For this review, take the finished solid that the model builds, in its own axes (mm). A direction names the side the tool comes from. Round coordinates to 2 decimals unless told otherwise and drop trailing zeros. Order: outer loops, then holes, each group sorted by start corner. A loop starts at its lowest first (then second) coordinate and runs counter-clockwise, first axis right, second up. Notation, with made-up numbers: (-37, -37.75) -> (4, -37.75) arc R18 cw to (4, -6.75) -> close; hole circle Ø4 at (55, -3.5). An arc over 180 degrees is marked (long way). Use a Markdown table: item, result. Add a question column.
1) Draft analysis for pull direction Y (two halves, no side actions). For faces 5 (the face through (9, -2.54, 64)), 6 (the face through (10, 4, 25.4)), 7 (the face through (14.188, 4, 15)), state which applies: pulls with the +Y half, pulls with the -Y half, needs draft (parallel to the pull), parting line crosses it, or undercut.
2) Machinability: for faces 1 (the face through (13.31, 5.03, 12.52)), 2 (the face through (19.05, -1, 56)), 3 (the face through (10, 4, 30.48)), 4 (the face through (6.568, 4, 15)), which of the approach directions +Z, -Z, +X, -X, +Y, -Y give a long, thin tool a straight path to every point of the face, cutting with its end or side? Answer none if there is none.
3) Consider section D-D (y = -1.25). State the section outline as (x, z) points (3 decimals), plus the area to 3 significant figures.
4) Wall thickness on line 1 along X through (y, z) = (3.81, 18); line 2 along Y through (x, z) = (13, 40); line 3 along Y through (x, z) = (10.25, 23.5): over which ranges is each line inside the solid? List them lowest first. Write a range as [from, to].
5) Clearance check with flat-ended pins moving along their axes: P1, Ø5, axis at x = 11.5, y = 3.5, coming from the -Z side; P2, Ø4, axis at x = 10.38, y = 3.81, coming from the -Z side; P3, Ø4, axis at x = 13.5, y = 5.5, coming from the +Z side; P4, Ø10, axis at x = 15.5, z = 92, coming from the +Y side. State where each tip first meets the part, or that it passes through.
6) Consider section A-A (z = 26.5). State the section outline as (x, y) points, plus the area to 3 significant figures.
7) Consider section C-C (x = 11). State the section outline as (y, z) points, plus the area to 3 significant figures.
8) Consider section B-B (y = 3.81). State the section outline as (x, z) points.
```python
from build123d import *

# Parameters (mm, degrees)
F1_DEPTH = 2.54
F2_W     = 7.62
F2_H     = 30.48
F3_DEPTH = 7.62
F4_R     = 3.175
F5_DEPTH = 25.4


with BuildPart() as f1:
    # F0 (on Front) → F1 (new body)
    with BuildSketch(Plane.XZ):
        Polygon((0, 114.3), (0, 0), (19.05, 0), (19.05, 114.3), (9.525, 127), align=None)
    extrude(amount=F1_DEPTH)

    # F2 (on face) → F3 (join)
    with BuildSketch(Plane(origin=(0, 0, 0), x_dir=(-1, 0, 0), z_dir=(0, 1, 0))):
        with Locations((-10.377643, 15.24)):
            Rectangle(F2_W, F2_H)
    extrude(amount=F3_DEPTH)

    # F4 (on face) → F5 (cut)
    with BuildSketch(Plane(origin=(0, 0, 0), x_dir=(1, 0, 0), z_dir=(0, 0, -1))):
        with Locations((10.377643, -3.81)):
            Circle(F4_R)
    extrude(amount=-F5_DEPTH, mode=Mode.SUBTRACT)


solid = f1.part
```
Results list:
| question | item | result |
|---|---|---|
| 1 | face 5 | pulls with the -Y half |
| 1 | face 6 | undercut |
| 1 | face 7 | needs draft |
| 2 | face 1 | -Z |
| 2 | face 2 | +Z, -Z, +X, +Y, -Y |
| 2 | face 3 | +Z, +X, -X, +Y |
| 2 | face 4 | +Z, -Z, -X, +Y |
| 3 | outline | (0, 0) -> (19.05, 0) -> (19.05, 114.3) -> (9.525, 127) -> (0, 114.3) -> close |
| 3 | area | 2,300 mm2 |
| 4 | line 1 | [6.57, 7.2], [13.55, 14.19] |
| 4 | line 2 | [-2.54, 0] |
| 4 | line 3 | [-2.54, 0.64], [6.98, 7.62] |
| 5 | P1 | z = 0 |
| 5 | P2 | z = 25.4 |
| 5 | P3 | z = 30.48 |
| 5 | P4 | y = 0 |
| 6 | outline | (0, -2.54) -> (19.05, -2.54) -> (19.05, 0) -> (14.19, 0) -> (14.19, 7.62) -> (6.57, 7.62) -> (6.57, 0) -> (0, 0) -> close |
| 6 | area | 106 mm2 |
| 7 | outline | (-2.54, 0) -> (0.7, 0) -> (0.7, 25.4) -> (6.92, 25.4) -> (6.92, 0) -> (7.62, 0) -> (7.62, 30.48) -> (0, 30.48) -> (0, 125.03) -> (-2.54, 125.03) -> close |
| 7 | area | 392 mm2 |
| 8 | outline | (6.57, 0) -> (7.2, 0) -> (7.2, 25.4) -> (13.55, 25.4) -> (13.55, 0) -> (14.19, 0) -> (14.19, 30.48) -> (6.57, 30.48) -> close |
